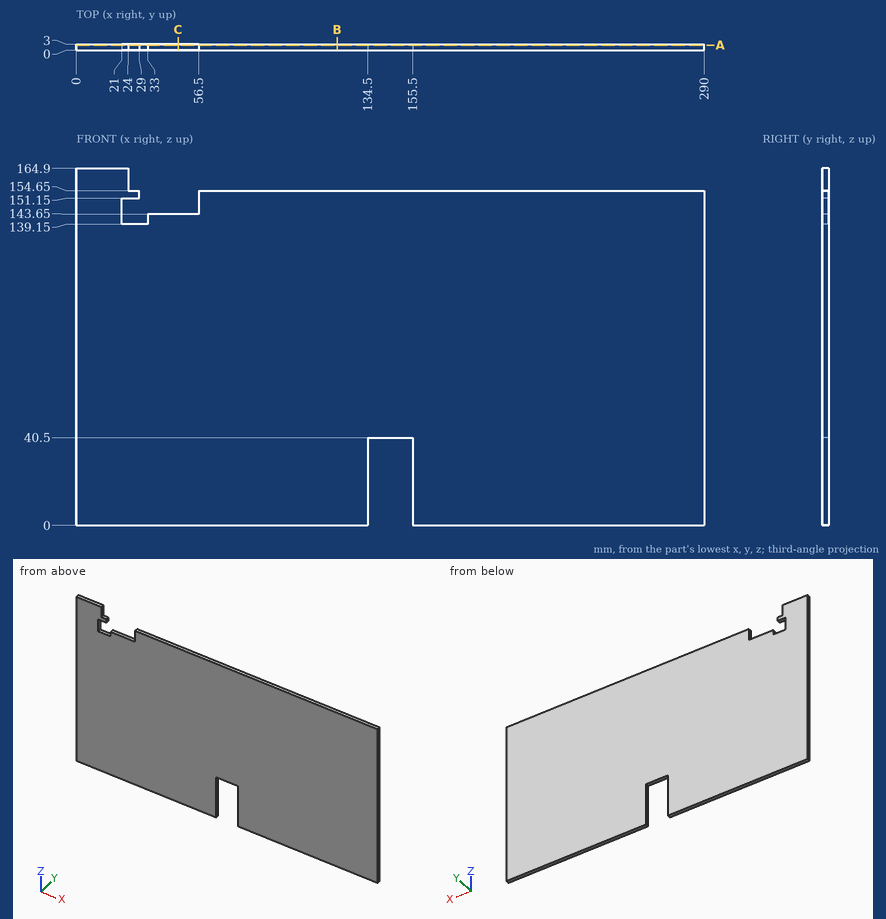
Could you check a few things on this drawing? It's one solid part, dimensions in mm from its lowest x, y, z. Coordinates: 2 decimals unless noted, no trailing zeros. Write each loop counter-clockwise with the first axis right and the second up, starting at its lowest first coordinate (ties: lowest second). Pieces come first, ordered by that corner, then holes. Notation, with made-up numbers: (60.5, 82.25) - (90.5, 82.25) arc R21 ccw to (90.5, 119.25) - close; hole circle Ø6 at (1.5, -34). An arc over 180 degrees is marked (long way). Return JSON: item names as keys, results as strings. Group by question number.
Item 1: If we section it at A-A (y = 2.45): Write out the boundary of the cut face in (x, z), then the cut area to 3 significant figures.
Item 2: If we section it at C-C (x = 47): Write out the boundary of the cut face in (y, z).
Item 3: If we section it at B-B (x = 120.5): Write out the boundary of the cut face in (y, z), then the cut area to 3 significant figures.
Item 4: I'm going to push flat-ended pins straight in: pin 1 Ø1 at (x, y) = (43, 2) entering from +Z; pin 2 Ø1.5 at (y, z) = (1.5, 157.5) entering from +X; pin 3 Ø0.9 at (x, y) = (157.5, 2) entering from +Z. Where does each tip first touch, or does it pass through?
Item 5: Please list where these lines run through material, in increasing order: probe 1 along X at (y, z) = (1.1, 26.5); probe 2 along X at (y, z) = (2.3, 153.5); probe 3 along Z at (x, y) = (202, 2.85).
Return value:
{
 "1": {"outline": "(0, 0) - (134.5, 0) - (134.5, 40.5) - (155.5, 40.5) - (155.5, 0) - (290, 0) - (290, 154.65) - (56.5, 154.65) - (56.5, 143.65) - (33, 143.65) - (33, 139.15) - (21, 139.15) - (21, 151.15) - (29, 151.15) - (29, 154.65) - (24, 154.65) - (24, 164.9) - (0, 164.9) - close", "area": "43,800 mm^2"},
 "2": {"outline": "(0, 0) - (3, 0) - (3, 143.65) - (0, 143.65) - close"},
 "3": {"outline": "(0, 0) - (3, 0) - (3, 154.65) - (0, 154.65) - close", "area": "464 mm^2"},
 "4": {"pin 1": "stops at z = 143.65", "pin 2": "stops at x = 24", "pin 3": "stops at z = 154.65"},
 "5": {"probe 1": "x = 0 to 134.5, 155.5 to 290", "probe 2": "x = 0 to 29, 56.5 to 290", "probe 3": "z = 0 to 154.65"}
}
